Design review of the part built by this model. Coordinates are the model's own, in mm. A direction names the side the tool comes from. Coordinates: 2 decimals unless noted, no trailing zeros. Order: outer loops, then holes, each group sorted by start corner. A loop starts at its lowest first (then second) coordinate and runs counter-clockwise, first axis right, second up. Notation, with made-up numbers: (8.5, 33.5) -> (41.5, 33.5) arc R35 ccw to (41.5, 65.5) -> close; hole circle Ø5 at (46, 21). An arc over 180 degrees is marked (long way). Write item = value, one per line.
```python
from build123d import *

# Parameters (mm, degrees)
SKETCH1_R                    = 5
DRIVELINE_AXIS_DEPTH         = 23
DUMMY_BOSS_DEPTH             = 26
PIN_BASE_DEPTH               = 44
PIN_HOLES_D                  = 3.4
SKETCH8_R                    = 1.5
UPRIGHTS_DEPTH               = 10
UPRIGHTS_DEPTH_BACK          = 3
SKETCH9_R                    = 1.5
SHOCK_MOUNT_DEPTH            = 5
SHOCK_MOUNT_DEPTH_BACK       = 13
SKETCH10_R                   = 1.5
TURNBUCKLE_MOUNTS_DEPTH      = 3
TURNBUCKLE_MOUNTS_DEPTH_BACK = 6
TURNBUCKLE_ROOM_DEPTH        = 1
TURNBUCKLE_ROOM_DEPTH_BACK   = 23
ARM_PROFILE_R                = 4.5
CHASSIS_MOUNT_DEPTH          = 7
SKETCH29_W                   = 17.866942734
SKETCH29_H                   = 5.34009454
TRIM_DEPTH                   = 50
SKETCH30_R                   = 2
CHASSIS_HOLES_DEPTH          = 7
BOSS_EXTRUDE2_DEPTH          = 12.5
BOSS_EXTRUDE3_DEPTH          = 3
SKETCH43_R                   = 2.5
BOSS_EXTRUDE4_DEPTH          = 24
SKETCH45_W                   = 10.988682225
SKETCH45_H                   = 8
CUT_EXTRUDE5_DEPTH           = 14


with BuildPart() as part:
    # Sketch1 → Driveline Axis (new body, symmetric)
    with BuildSketch(Plane(origin=(0, 0, 0), x_dir=(0, 0, -1), z_dir=(1, 0, 0))):
        Circle(SKETCH1_R)
    extrude(amount=DRIVELINE_AXIS_DEPTH, both=True)

    # Sketch2 → Dummy Boss (add, symmetric)
    with BuildSketch(Plane.XY):
        Polygon((-12.5, -20), (-12.5, 14.464466094), (-8.964466094, 18), (8.964466094, 18), (12.5, 14.464466094), (12.5, -20), align=None)
    extrude(amount=DUMMY_BOSS_DEPTH, both=True)

    # Sketch3 → Pin Base (add)
    with BuildSketch(Plane(origin=(0, 0, -18), x_dir=(-1, 0, 0), z_dir=(0, 0, -1))):
        with BuildLine():
            Line((-19.5, -23), (19.5, -23))
            Line((19.5, -23), (24.664120213, -20.637403458))
            ThreePointArc((24.664120213, -20.637403458), (26.637403458, -15.335879787), (21.335879787, -13.362596542))
            Line((21.335879787, -13.362596542), (14.5, -16.490026826))
            Line((14.5, -16.490026826), (12.5, -16.490026826))
            Line((12.5, -16.490026826), (12.5, -20))
            Line((12.5, -20), (-12.5, -20))
            Line((-12.5, -20), (-12.5, -16.490026826))
            Line((-12.5, -16.490026826), (-14.5, -16.490026826))
            Line((-14.5, -16.490026826), (-21.335879787, -13.362596542))
            ThreePointArc((-21.335879787, -13.362596542), (-26.637403458, -15.335879787), (-24.664120213, -20.637403458))
            Line((-24.664120213, -20.637403458), (-19.5, -23))
        make_face()
    extrude(amount=-PIN_BASE_DEPTH)

    # Pin Holes (through all)
    with Locations(Plane(origin=(0, 0, -18), x_dir=(-1, 0, 0), z_dir=(0, 0, -1))):
        with Locations((-23, -17), (23, -17)):
            Hole(PIN_HOLES_D / 2)

    # Sketch8 → Uprights (add, two sides)
    with BuildSketch(Plane.XY) as uprights_sk:
        with BuildLine():
            Line((-10.732233047, 16.232233047), (-24.661465898, 46.103569293))
            Line((-24.661465898, 46.103569293), (-33.048979486, 47.815663334))
            ThreePointArc((-33.048979486, 47.815663334), (-35.583316151, 51.65), (-31.748979486, 54.184336666))
            Line((-31.748979486, 54.184336666), (-6.351020514, 49))
            Line((-6.351020514, 49), (6.351020514, 49))
            Line((6.351020514, 49), (31.748979486, 54.184336666))
            ThreePointArc((31.748979486, 54.184336666), (35.583316151, 51.65), (33.048979486, 47.815663334))
            Line((33.048979486, 47.815663334), (24.661465898, 46.103569293))
            Line((24.661465898, 46.103569293), (10.732233047, 16.232233047))
            Line((10.732233047, 16.232233047), (8.964466094, 18))
            Line((8.964466094, 18), (-8.964466094, 18))
            Line((-8.964466094, 18), (-10.732233047, 16.232233047))
        make_face()
        with Locations((-27.5, 50)):
            Circle(SKETCH8_R, mode=Mode.SUBTRACT)
        with Locations((27.5, 50)):
            Circle(SKETCH8_R, mode=Mode.SUBTRACT)
        with BuildLine():
            Line((9.866245938, 21.994232403), (1.612099151, 32.1872548))
            Line((1.612099151, 32.1872548), (22.924030195, 47.110029571))
            Line((22.924030195, 47.110029571), (10.997739753, 21.534017182))
            ThreePointArc((10.997739753, 21.534017182), (10.467987263, 21.852621345), (9.866245938, 21.994232403))
        make_face(mode=Mode.SUBTRACT)
        with BuildLine():
            Line((7.714466094, 20), (-7.714466094, 20))
            ThreePointArc((-7.714466094, 20), (-7.795487149, 20.563488959), (-8.031985901, 21.081323449))
            Line((-8.031985901, 21.081323449), (0, 31))
            Line((0, 31), (8.031985901, 21.081323449))
            ThreePointArc((8.031985901, 21.081323449), (7.795487149, 20.563488959), (7.714466094, 20))
        make_face(mode=Mode.SUBTRACT)
        with BuildLine():
            Line((-10.997739753, 21.534017182), (-22.924030195, 47.110029571))
            Line((-22.924030195, 47.110029571), (-1.612099151, 32.1872548))
            Line((-1.612099151, 32.1872548), (-9.866245938, 21.994232403))
            ThreePointArc((-9.866245938, 21.994232403), (-10.467987263, 21.852621345), (-10.997739753, 21.534017182))
        make_face(mode=Mode.SUBTRACT)
        Polygon((-19.279998091, 47), (0, 33.5), (19.279998091, 47), align=None, mode=Mode.SUBTRACT)
    extrude(amount=UPRIGHTS_DEPTH)
    extrude(uprights_sk.sketch, amount=-UPRIGHTS_DEPTH_BACK)

    # Sketch9 → Shock Mount (add, two sides)
    with BuildSketch(Plane.XY.offset(10)) as shock_mount_sk:
        with BuildLine():
            Line((-24.661465898, 46.103569293), (-33.048979486, 47.815663334))
            ThreePointArc((-33.048979486, 47.815663334), (-35.583316151, 51.65), (-31.748979486, 54.184336666))
            Line((-31.748979486, 54.184336666), (-23.361465898, 52.472242624))
            ThreePointArc((-23.361465898, 52.472242624), (-20.827129232, 48.637905958), (-24.661465898, 46.103569293))
        make_face()
        with Locations((-27.5, 50)):
            Circle(SKETCH9_R, mode=Mode.SUBTRACT)
        with BuildLine():
            Line((23.361465898, 52.472242624), (31.748979486, 54.184336666))
            ThreePointArc((31.748979486, 54.184336666), (35.583316151, 51.65), (33.048979486, 47.815663334))
            Line((33.048979486, 47.815663334), (24.661465898, 46.103569293))
            ThreePointArc((24.661465898, 46.103569293), (20.827129232, 48.637905958), (23.361465898, 52.472242624))
        make_face()
        with Locations((27.5, 50)):
            Circle(SKETCH9_R, mode=Mode.SUBTRACT)
    extrude(amount=SHOCK_MOUNT_DEPTH)
    extrude(shock_mount_sk.sketch, amount=-SHOCK_MOUNT_DEPTH_BACK)

    # Sketch10 → Turnbuckle Mounts (add, two sides)
    with BuildSketch(Plane.XY) as turnbuckle_mounts_sk:
        with BuildLine():
            Line((29.5, 8), (12.5, 8))
            Line((12.5, 8), (12.5, 14.464466094))
            Line((12.5, 14.464466094), (21.055616084, 16.739249053))
            ThreePointArc((21.055616084, 16.739249053), (22.124817677, 17.666247097), (23.5, 18))
            Line((23.5, 18), (29.5, 18))
            ThreePointArc((29.5, 18), (31.621320344, 17.121320344), (32.5, 15))
            Line((32.5, 15), (32.5, 11))
            ThreePointArc((32.5, 11), (31.621320344, 8.878679656), (29.5, 8))
        make_face()
        with Locations((23.5, 11)):
            Circle(SKETCH10_R, mode=Mode.SUBTRACT)
        with BuildLine():
            Line((-12.5, 14.464466094), (-21.055616084, 16.739249053))
            ThreePointArc((-21.055616084, 16.739249053), (-22.124817677, 17.666247097), (-23.5, 18))
            Line((-23.5, 18), (-29.5, 18))
            ThreePointArc((-29.5, 18), (-31.621320344, 17.121320344), (-32.5, 15))
            Line((-32.5, 15), (-32.5, 11))
            ThreePointArc((-32.5, 11), (-31.621320344, 8.878679656), (-29.5, 8))
            Line((-29.5, 8), (-12.5, 8))
            Line((-12.5, 8), (-12.5, 14.464466094))
        make_face()
        with Locations((-23.5, 11)):
            Circle(SKETCH10_R, mode=Mode.SUBTRACT)
    extrude(amount=TURNBUCKLE_MOUNTS_DEPTH)
    extrude(turnbuckle_mounts_sk.sketch, amount=-TURNBUCKLE_MOUNTS_DEPTH_BACK)

    # Sketch11 → Turnbuckle Room (cut, two sides)
    with BuildSketch(Plane(origin=(0, 0, -26), x_dir=(-1, 0, 0), z_dir=(0, 0, -1))) as turnbuckle_room_sk:
        Polygon((8.964466094, 18), (5.75, 18), (5.75, 8), (12.5, 1.544903812), (12.5, 14.464466094), align=None)
        Polygon((-12.5, 14.464466094), (-12.5, 1.464466094), (-6.25, 8), (-6.25, 18), (-8.964466094, 18), align=None)
    extrude(amount=TURNBUCKLE_ROOM_DEPTH, mode=Mode.SUBTRACT)
    extrude(turnbuckle_room_sk.sketch, amount=-TURNBUCKLE_ROOM_DEPTH_BACK, mode=Mode.SUBTRACT)

    # Arm: sweep along a path in Sketch13
    with BuildLine(Plane(origin=(14.391793376, 0, 5.313892939), x_dir=(0.346374083, 0, -0.938096474), z_dir=(0.938096474, 0, 0.346374083))) as arm_path:
        Line((24.852340438, -17), (84.852340438, 13))
    # Arm profile (on start of the path) → Arm (sweep)
    with BuildSketch(Plane(origin=(23, -17, -18), x_dir=(0, -0.88247717, -0.470355232), z_dir=(0.309806398, 0.447213595, -0.839058994))):
        Circle(ARM_PROFILE_R)
    arm = sweep(path=arm_path.line)

    # Mirror1: Arm across plane
    add(arm.mirror(Plane(origin=(0, 0, 0), x_dir=(0, 0, 1), z_dir=(1, 0, 0))))

    # Sketch28 → Chassis mount (add)
    with BuildSketch(Plane(origin=(0, 13, 0), x_dir=(-1, 0, 0), z_dir=(0, -1, 0))):
        with BuildLine():
            Line((-39.282444966, 74.285788448), (-39.282444966, 68.285788448))
            Line((-39.282444966, 68.285788448), (-48.282444966, 68.285788448))
            Line((-48.282444966, 68.285788448), (-48.282444966, 74.285788448))
            ThreePointArc((-48.282444966, 74.285788448), (-43.782444966, 78.785788448), (-39.282444966, 74.285788448))
        make_face()
    chassis_mount = extrude(amount=CHASSIS_MOUNT_DEPTH)

    # Mirror2: Chassis mount across plane
    add(chassis_mount.mirror(Plane(origin=(0, 0, 0), x_dir=(0, 0, 1), z_dir=(1, 0, 0))))

    # Sketch29 → Trim (cut, symmetric)
    with BuildSketch(Plane(origin=(0, 0, 0), x_dir=(0, 0, -1), z_dir=(1, 0, 0))):
        with Locations((69.852317081, 15.67004727)):
            Rectangle(SKETCH29_W, SKETCH29_H)
    extrude(amount=TRIM_DEPTH, both=True, mode=Mode.SUBTRACT)

    # Sketch30 → Chassis Holes (cut)
    with BuildSketch(Plane(origin=(0, 13, 0), x_dir=(-1, 0, 0), z_dir=(0, -1, 0))):
        with Locations((-43.782444966, 74.285788448)):
            Circle(SKETCH30_R)
    chassis_holes = extrude(amount=CHASSIS_HOLES_DEPTH, mode=Mode.SUBTRACT)

    # Mirror3: Chassis Holes across plane
    add(chassis_holes.mirror(Plane(origin=(0, 0, 0), x_dir=(0, 0, 1), z_dir=(1, 0, 0))), mode=Mode.SUBTRACT)

    # Sketch40 → Boss-Extrude2 (add, symmetric)
    with BuildSketch(Plane(origin=(0, 0, 0), x_dir=(0, 0, -1), z_dir=(1, 0, 0))):
        Polygon((26, -13.545257512), (39.035885991, -6.100654803), (56.964114009, -3.899345197), (56.964114009, -6.921874674), (40, -9.004805964), (26, -17), align=None)
    extrude(amount=BOSS_EXTRUDE2_DEPTH, both=True)

    # Sketch41 → Boss-Extrude3 (add)
    with BuildSketch(Plane(origin=(0, -10.73186481, -1.317707308), x_dir=(1, 0, 0), z_dir=(0, 0.992546152, 0.121869343))):
        with BuildLine():
            Line((12.5, 56.064301503), (12.5, 38.001435621))
            ThreePointArc((12.5, 38.001435621), (21.531432941, 47.032868562), (12.5, 56.064301503))
        make_face()
    boss_extrude3 = extrude(amount=-BOSS_EXTRUDE3_DEPTH)

    # Mirror4: Boss-Extrude3 across plane
    add(boss_extrude3.mirror(Plane(origin=(0, 0, 0), x_dir=(0, 0, 1), z_dir=(1, 0, 0))))

    # Sketch43 → Boss-Extrude4 (add)
    with BuildSketch(Plane(origin=(0, -10.73186481, -1.317707308), x_dir=(1, 0, 0), z_dir=(0, 0.992546152, 0.121869343))):
        with Locations((-15, 47.032868562)):
            Circle(SKETCH43_R)
        with Locations((15, 47.032868562)):
            Circle(SKETCH43_R)
    extrude(amount=BOSS_EXTRUDE4_DEPTH)

    # Sketch45 → Cut-Extrude5 (cut)
    with BuildSketch(Plane.XZ.offset(23)):
        with Locations((24.994341113, -14)):
            Rectangle(SKETCH45_W, SKETCH45_H)
        with Locations((24.994341113, 24)):
            Rectangle(SKETCH45_W, SKETCH45_H)
        with Locations((-24.994341113, 24)):
            Rectangle(SKETCH45_W, SKETCH45_H)
        with Locations((-24.994341113, -14)):
            Rectangle(SKETCH45_W, SKETCH45_H)
    extrude(amount=-CUT_EXTRUDE5_DEPTH, mode=Mode.SUBTRACT)


solid = part.part
```
(1) For L1, parallel to X at y = 38, z = 8; L2, parallel to Y at x = -23, z = 12; L3, parallel to X at y = -14, z = -12, list the stretches that pass through material, from the lowest coordinate up.
Report:
L1 = -20.88 to -18.68, -9.91 to -6.43, 6.43 to 9.91, 18.68 to 20.88
L2 = -21.4 to -18.7, -15.3 to -13, 46.2 to 52.38
L3 = -12.5 to 12.5
(2) The part is to be moulded in two halves that separate along X. For faces 5 (the flat face through (-23, 0, 0)), 6 (the flat face through (0, 18, -14)), 7 (the cylindrical face through (22.11, 17.66, -1.44)), say which applies: released by +X, released by -X, zero draft, split by the parting line, or undercut.
Report:
face_5 = released by -X
face_6 = zero draft
face_7 = undercut
(3) We need section A-A (z = -7.5). Write out the cut boundary in (x, y).
Report:
outline = (-24.66, -20.64) -> (-19.5, -23) -> (19.5, -23) -> (24.66, -20.64) arc R4 ccw to (21.34, -13.36) -> (14.5, -16.49) -> (12.5, -16.49) -> (12.5, 1.46) -> (6.25, 8) -> (6.25, 18) -> (-5.75, 18) -> (-5.75, 8) -> (-12.5, 1.54) -> (-12.5, -16.49) -> (-14.5, -16.49) -> (-21.34, -13.36) arc R4 ccw to start; hole circle Ø3.4 at (-23, -17); hole circle Ø3.4 at (23, -17)
(4) For faces 1 (the flat face through (39.282, 7, -73)), 2 (the flat face through (-23, 13, 3)), 3 (the flat face through (23, 0, 0)), 4 (the flat face through (-26, 18, -2)), list the 3-axis set-ups (+Z, -Z, +X, -X, +Y, -Y) from which the entire face can be reached by the end or side of a thin tool; tool diameter is ignored.
Report:
face_1 = -Z, -Y
face_2 = +Z, -X
face_3 = +Z, -Z, +X
face_4 = +Z, -Z, -X
(5) Insertion check: pin 1 (14.5 mm diameter, centred on x = -1, z = 1, fed in from +Y); pin 2 (8 mm diameter, centred on x = -7, z = 1, fed in from +Y); pin 3 (8 mm diameter, centred on y = 25.5, z = -48, fed in from -X); pin 4 (5 mm diameter, centred on x = -27.5, y = 50, fed in from -Z). Each pin has a flat end and moves straight along its axis. Give the tip position at first contact, or say it passes through.
Report:
pin_1 = 49.39
pin_2 = 49.95
pin_3 = through
pin_4 = -3
(6) We need section B-B (x = -4). Write out the cut boundary in (y, z).
Report:
outline = (-23, -18) -> (-20, -18) -> (-20, -26) -> (-17, -26) -> (-9, -40) -> (-6.92, -56.96) -> (-3.9, -56.96) -> (-6.1, -39.04) -> (-13.55, -26) -> (18, -26) -> (18, -3) -> (20, -3) -> (20, 10) -> (18, 10) -> (18, 26) -> (-23, 26) -> close; (26.06, -3) -> (29.24, -3) -> (29.24, 10) -> (26.06, 10) -> close; (33.86, -3) -> (36.3, -3) -> (36.3, 10) -> (33.86, 10) -> close; (47, -3) -> (49, -3) -> (49, 10) -> (47, 10) -> close
(7) We need section D-D (z = 17.5). Write out the cut boundary in (x, y).
Report:
outline = (-24.66, -20.64) -> (-19.5, -23) -> (19.5, -23) -> (24.66, -20.64) arc R4 ccw to (21.34, -13.36) -> (14.5, -16.49) -> (12.5, -16.49) -> (12.5, 14.46) -> (8.96, 18) -> (-8.96, 18) -> (-12.5, 14.46) -> (-12.5, -16.49) -> (-14.5, -16.49) -> (-21.34, -13.36) arc R4 ccw to start; hole circle Ø3.4 at (-23, -17); hole circle Ø3.4 at (23, -17)
(8) We need section C-C (y = 28). Write out the cut boundary in (x, z).
Report:
outline = (-16.22, -3) -> (-14.01, -3) -> (-14.01, 10) -> (-16.22, 10) -> close; (-5, -3) -> (-2.43, -3) -> (-2.43, 10) -> (-5, 10) -> close; (2.43, -3) -> (5, -3) -> (5, 10) -> (2.43, 10) -> close; (14.01, -3) -> (16.22, -3) -> (16.22, 10) -> (14.01, 10) -> close
